Geometry: final body of the model. Coordinates: model frame, mm. Face numbers are marked on the shaded views. A direction names the side the tool comes from. Give positions to 0.01 mm unless a question says otherwise; leave off trailing zeros. Write each loop counter-clockwise with the first axis right and the second up, starting at its lowest first coordinate (ties: lowest second). Pieces come first, ordered by that corner, then holes. Notation, with made-up numbers: (-1.75, -22.75) - (10.25, -22.75) arc R24 cw to (10.25, 14.25) - close; hole circle Ø5 at (35, 26). An arc over 180 degrees is marked (long way). Use CSV: the item, a comma, the result in double quotes. Start each with the question number.
(1) Draft query along X for the marked faces 4, 5, 6 and 7. Return one class per face: released by +X, released by -X, zero draft, split by the parting line, or undercut.
(2) Section A-A on x = 2. Output: boundary loops of the cut face in (y, z), and give its area (3 significant figures).
(3) Section B-B on z = 7. Output: boundary loops of the cut face in (x, y), and give its area (3 significant figures).
(4) Reachability of the marked faces 1, 2 and 3 from +Z, -Z, +X, -X, +Y, -Y: full face, straight path, thin tool, end or side. Return the list, or none.
(5) Line query: probe 1 along Z at (x, y) = (-16.5, 5.75); probe 2 along Z at (x, y) = (-12, 7.25); probe 3 along X at (y, z) = (4.5, 13). Output: solid intervals per line, ascending. Write a range as [from, to].
(6) First-contact query: pin 1 Ø2 at (y, z) = (3.5, -15.5) entering from +X; pin 2 Ø1 at (x, y) = (-7, 5.5) entering from -Z; pin 3 Ø4 at (x, y) = (15, 5) entering from -Z. Flat tips, straight axial feed; report the tip coordinate or a pass-through.
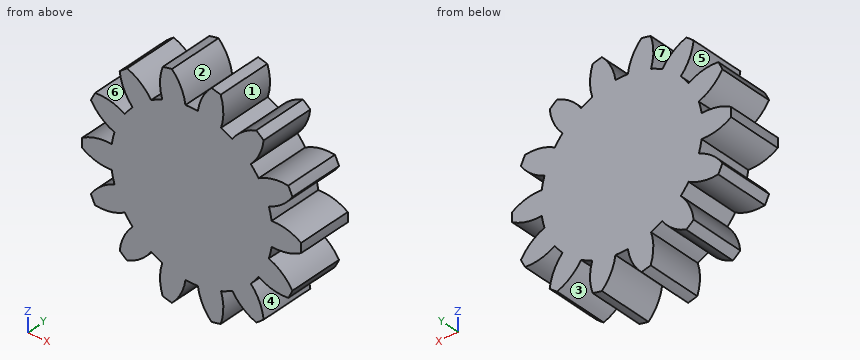
from build123d import *

# Parameters (mm, degrees)
SKETCH_1_R               = 20
EXTRUDE_1_DEPTH          = 10
CUT_EXTRUDE_1_DEPTH      = 31
PATTERN_CIRCULAR_1_COUNT = 14


with BuildPart() as part:
    # 草图1 → 凸台-拉伸1 (new body)
    with BuildSketch(Plane(origin=(0, 0, 0), x_dir=(1, 0, 0), z_dir=(0, 1, 0))):
        with Locations(Location((0, 0, 0), (0, 0, 270))):
            Circle(SKETCH_1_R)
    extrude(amount=EXTRUDE_1_DEPTH)

    # 草图2 → 切除-拉伸1 (cut, symmetric)
    with BuildSketch(Plane(origin=(0, 10, 0), x_dir=(1, 0, 0), z_dir=(0, 1, 0))):
        with BuildLine():
            ThreePointArc((-1.13256244, 14.706454444), (0, 14.75), (1.13256244, 14.706454444))
            ThreePointArc((1.13256244, 14.706454444), (1.960472225, 17.392163769), (3.60273366, 19.672831778))
            ThreePointArc((3.60273366, 19.672831778), (0, 20), (-3.60273366, 19.672831778))
            ThreePointArc((-3.60273366, 19.672831778), (-1.960472225, 17.392163769), (-1.13256244, 14.706454444))
        make_face()
    cut_extrude_1 = extrude(amount=CUT_EXTRUDE_1_DEPTH, both=True, mode=Mode.SUBTRACT)

    # 阵列(圆周)1: 切除-拉伸1 ×14 about axis
    pattern_circular_1_axis = Axis((0, 0, 0), (0, 1, 0))
    for i in range(1, PATTERN_CIRCULAR_1_COUNT):
        add(cut_extrude_1.rotate(pattern_circular_1_axis, i * 360 / PATTERN_CIRCULAR_1_COUNT), mode=Mode.SUBTRACT)


solid = part.part
Check values:
1,face 4,"released by +X"
1,face 5,"released by -X"
1,face 6,"undercut"
1,face 7,"undercut"
2,outline,"(0, -17.47) - (10, -17.47) - (10, 17.47) - (0, 17.47) - close"
2,area,"349 mm²"
3,outline,"(-17.74, 0) - (17.74, 0) - (17.74, 10) - (-17.74, 10) - close"
3,area,"355 mm²"
4,face 1,"+Y, -Y"
4,face 2,"+Z, +Y, -Y"
4,face 3,"-Z, +Y, -Y"
5,probe 1,"z = [-9.5, -5.77], [-2.13, 2.13], [5.77, 9.5]"
5,probe 2,"z = [-16, -11.66], [-8.58, 8.58], [11.66, 16]"
5,probe 3,"x = [-12.64, -7.57], [-6.97, 6.97], [7.57, 12.64]"
6,pin 1,"stops at x = 13.13"
6,pin 2,"stops at z = -13.24"
6,pin 3,"stops at z = -15.2"
